Here's how the part is built. I have some questions about the finished solid (model axes, mm). A direction names the side the tool comes from. Coordinates: 2 decimals unless noted, no trailing zeros. Loops run counter-clockwise (first coordinate to the right, second up) from the corner with the lowest first, then second, coordinate; pieces in that order, holes last.
Autodesk Inventor part; units mm, degrees
ref_plane "2mm deep in well" through (0, 2, 0) normal (0, -1, 0) x (1, 0, 0)
ref_plane "YZ Plane" through (0, 0, 0) normal (1, 0, 0) x (0, 1, 0)
ref_plane "XZ Plane" through (0, 0, 0) normal (0, 1, 0) x (-1, 0, 0)
sketch "Sketch1" plane through (0, 0, 0) normal (0, 1, 0) x (-1, 0, 0)
  circle A0 centre (0, 0) radius 2.375
  circle A1 centre (0, 0) radius 3.45
  dimension "d0" = 4.75
  dimension "d1" = 6.9
extrude "Extrusion1" add sketch "Sketch1" along normal blind 3.75
ref_plane "2mm deep in well" through (0, 2, 0) normal (0, -1, 0) x (1, 0, 0)
sketch "Sketch2" plane through (0, 2, 0) normal (0, -1, 0) x (1, 0, 0)
  point P0 (0, 0)
sketch "Sketch3" plane through (0, 2, 0) normal (0, -1, 0) x (1, 0, 0)
  circle A0 centre (0, 0) radius 3.45
  circle A1 centre (0, 0) radius 2.375
  circle A2 centre (0, 0) radius 1.215
  dimension "d5" = 2.43
extrude "Extrusion2" add sketch "Sketch3" against normal blind 0.63 contours A1
sketch "Sketch4" plane through (0, 3.75, 0) normal (0, 1, 0) x (1, 0, 0)
  line L0 (-16, 0) -> (16, 0)
  circle A0 centre (14.075, 0) radius 1.925
  circle A1 centre (0, 0) radius 3.45
  circle A2 centre (0, 0) radius 2.375
  line L1 (2.221, 2.64) -> (2.221, -2.64)
  line L2 (2.221, 2.64) -> (14.075, 1.925)
  line L3 (2.221, -2.64) -> (14.075, -1.925)
  dimension "d8" = 32
  dimension "d9" = 0
  dimension "d10" = 0
  dimension "d11" = 3.85
  dimension "d12" = 1.925
  dimension "d13" = 0
  dimension "d14" = 5.28
extrude "Extrusion3" add sketch "Sketch4" against normal blind 1.43 contours A1 L2 A0 L0 | L0 A0 L3 A1 | A0 L0 | L0 A0
sketch "Sketch5" plane through (0, 3.75, 0) normal (0, 1, 0) x (1, 0, 0)
  circle A0 centre (14.485, 0) radius 0.465
  arc A1 (2.221, 2.64) -> (2.221, -2.64) centre (0, 0) ccw
  line L0 (2.221, -2.64) -> (14.075, -1.925)
  arc A2 (14.075, -1.925) -> (14.075, 1.925) centre (14.075, 0) ccw
  line L1 (14.075, 1.925) -> (2.221, 2.64)
  circle A3 centre (0, 0) radius 2.375
  point P0 (16, 0)
  dimension "d17" = 0.93
  dimension "d18" = 0
  dimension "d19" = 1.515
extrude "Extrusion4" cut sketch "Sketch5" against normal up to surface (1.43 mm away) contours A0
pattern_linear "Rectangular Pattern1" count 6 spacing 1.98 along (-1, 0, 0) of "Extrusion4"
mirror "Mirror1" about plane through (0, 0, 0) normal (1, 0, 0) of "Extrusion3", "Extrusion4", "Rectangular Pattern1"
properties part number "Servo Horn"
Q1. Will these pins go through, and if not, where does the flat tip stop? P1, Ø1, axis at y = 1, z = 2.5, coming from the +X side; P2, Ø1.6, axis at x = -9, z = -1, coming from the -Y side; P3, Ø3, axis at x = 0, z = 0, coming from the +Y side.
Q2. Please list where these lines run through material, in increasing order: probe 1 along Z at (x, y) = (0, 1.9) (3 decimals); probe 2 along Y at (x, z) = (-12.5, -1.5); probe 3 along Z at (x, y) = (-8.5, 3.3).
Q3. Suppose I cut it at A-A on x = -8.5. Write out the boundary of the cut face in (y, z), and give its area (3 significant figures).
Q4. Suppose I cut it at C-C on z = -1.5. Write out the boundary of the cut face in (x, y).
Q5. We'd pull the mould along X, two halves only. Please class faces 4 (the flat face through (9, 2.32, 1)), 5 (the flat face through (-8.231, 3.045, -2.277)), 6 (the cylindrical face through (-14.93, 3.05, 0.14)): pulls with the +X half, pulls with the -X half, needs draft (parallel to the pull), parting line crosses it, or undercut.
Q6. Suppose I cut it at B-B on y = 1.55. Write out the boundary of the cut face in (x, z) (3 decimals), and give its area (3 significant figures).
Q7. For faces 1 (the flat face through (-1, 2.63, 1)), 2 (the flat face through (-8.231, 3.045, 2.277)), 3 (the cylindrical face through (-1.096, 0.986, 2.107)), which set-ups out of +Z, -Z, +X, -X, +Y, -Y let a thin tool reach every point of the face, with its end or its side?
Q8. Suppose I cut it at D-D on x = 0. Write out the boundary of the cut face in (y, z) (3 decimals).
Check values:
1. P1: stops at x = 2.81
1. P2: stops at y = 2.32
1. P3: stops at y = 2.63
2. probe 1: z = -3.45 to -2.375, 2.375 to 3.45
2. probe 2: y = 2.32 to 3.75
2. probe 3: z = -2.26 to -0.46, 0.46 to 2.26
3. outline: (2.32, -2.26) - (3.75, -2.26) - (3.75, -0.46) - (2.32, -0.46) - close; (2.32, 0.46) - (3.75, 0.46) - (3.75, 2.26) - (2.32, 2.26) - close
3. area: 5.14 mm2
4. outline: (-15.28, 2.32) - (-3.11, 2.32) - (-3.11, 0) - (-1.84, 0) - (-1.84, 2) - (1.84, 2) - (1.84, 0) - (3.11, 0) - (3.11, 2.32) - (15.28, 2.32) - (15.28, 3.75) - (1.84, 3.75) - (1.84, 2.63) - (-1.84, 2.63) - (-1.84, 3.75) - (-15.28, 3.75) - close
5. face 4: needs draft
5. face 5: pulls with the -X half
5. face 6: undercut
6. outline: circle Ø6.9 at (0, 0); hole circle Ø4.75 at (0, 0)
6. area: 19.7 mm2
7. face 1: +Y
7. face 2: +Z, -X, +Y, -Y
7. face 3: -Y
8. outline: (0, -3.45) - (3.75, -3.45) - (3.75, -2.375) - (2.63, -2.375) - (2.63, -1.215) - (2, -1.215) - (2, -2.375) - (0, -2.375) - close; (0, 2.375) - (2, 2.375) - (2, 1.215) - (2.63, 1.215) - (2.63, 2.375) - (3.75, 2.375) - (3.75, 3.45) - (0, 3.45) - close
